The model under review builds one solid part; all positions refer to its coordinate system, in mm. A direction names the side the tool comes from. Give positions to 0.01 mm unless a question says otherwise; leave off trailing zeros. Loops run counter-clockwise (first coordinate to the right, second up) from the corner with the lowest first, then second, coordinate; pieces in that order, holes last. Notation, with made-up numbers: M -23.5,-7 L 28.5,-7 A18 ccw 28.5,20 Z; hole C -7,11.25 d4. An arc over 180 degrees is marked long. Return JSON: item names as keys, results as strings. Group by question number.
```python
from build123d import *

# Parameters (mm, degrees)
SKETCH1_W           = 20
SKETCH1_H           = 18
BOSS_EXTRUDE1_DEPTH = 25
SKETCH2_R           = 4
CUT_EXTRUDE1_DEPTH  = 26
CHAMFER1_SIZE       = 2
BOSS_EXTRUDE2_DEPTH = 1.5
CUT_EXTRUDE2_DEPTH  = 0.5
BOSS_EXTRUDE3_DEPTH = 40
SKETCH6_W           = 1
SKETCH6_H           = 1
CUT_EXTRUDE3_DEPTH  = 8


with BuildPart() as part:
    # Sketch1 → Boss-Extrude1 (new body)
    with BuildSketch(Plane.XY):
        Rectangle(SKETCH1_W, SKETCH1_H)
    extrude(amount=BOSS_EXTRUDE1_DEPTH)

    # Sketch2 → Cut-Extrude1 (cut, through all)
    with BuildSketch(Plane.XY.offset(25)):
        Circle(SKETCH2_R)
    extrude(amount=-CUT_EXTRUDE1_DEPTH, mode=Mode.SUBTRACT)

    # Chamfer1
    chamfer1_edges = [part.edges().sort_by_distance(p)[0] for p in [
        (10, 9, 12.5),
        (10, -9, 12.5),
        (-10, -9, 12.5),
        (-10, 9, 12.5),
    ]]
    chamfer(chamfer1_edges, length=CHAMFER1_SIZE)

    # Sketch3 → Boss-Extrude2 (add)
    with BuildSketch(Plane(origin=(0, 9, 0), x_dir=(1, 0, 0), z_dir=(0, 1, 0))):
        with BuildLine():
            Line((-7.418918919, -22.013513514), (-1.418918919, -4.513513514))
            ThreePointArc((-1.418918919, -4.513513514), (0.486486486, -3.581081081), (1.418918919, -5.486486486))
            Line((1.418918919, -5.486486486), (-4.581081081, -22.986486486))
            ThreePointArc((-4.581081081, -22.986486486), (-6.486486486, -23.918918919), (-7.418918919, -22.013513514))
        make_face()
    extrude(amount=BOSS_EXTRUDE2_DEPTH)

    # Sketch4 → Cut-Extrude2 (cut)
    with BuildSketch(Plane(origin=(0, 10.5, 0), x_dir=(1, 0, 0), z_dir=(0, 1, 0))):
        with BuildLine():
            Line((-6.945945946, -22.175675676), (-0.945945946, -4.675675676))
            ThreePointArc((-0.945945946, -4.675675676), (0.324324324, -4.054054054), (0.945945946, -5.324324324))
            Line((0.945945946, -5.324324324), (-5.054054054, -22.824324324))
            ThreePointArc((-5.054054054, -22.824324324), (-6.324324324, -23.445945946), (-6.945945946, -22.175675676))
        make_face()
    extrude(amount=-CUT_EXTRUDE2_DEPTH, mode=Mode.SUBTRACT)

    # Sketch5 → Boss-Extrude3 (add)
    with BuildSketch(Plane(origin=(0, 0, 0), x_dir=(-1, 0, 0), z_dir=(0, 0, -1))):
        Polygon((-10, 4), (-16, 4), (-17, 3), (-17, -3), (-16, -4), (-10, -4), align=None)
    extrude(amount=-BOSS_EXTRUDE3_DEPTH)

    # Sketch6 → Cut-Extrude3 (cut, through all)
    with BuildSketch(Plane.ZY.offset(-10)):
        with Locations((25.5, 3.5)):
            Rectangle(SKETCH6_W, SKETCH6_H)
        with Locations((27.25, 3.5)):
            Rectangle(SKETCH6_W, SKETCH6_H)
        with Locations((29, 3.5)):
            Rectangle(SKETCH6_W, SKETCH6_H)
        with Locations((30.75, 3.5)):
            Rectangle(SKETCH6_W, SKETCH6_H)
    extrude(amount=-CUT_EXTRUDE3_DEPTH, mode=Mode.SUBTRACT)


solid = part.part
```
(1) Add section B-B (z = 2.5). Write out the cut boundary in (x, y), and give its area (3 significant figures).
(2) Add section C-C (x = 15). Write out the cut boundary in (y, z), and give its area (3 significant figures).
(3) Add section A-A (y = 0). Write out the cut boundary in (x, z).
(4) Add section D-D (z = 37.5). Write out the cut boundary in (x, y).
(5) For pin 1 (0.8 mm diameter, centred on x = 15, z = 27, fed in from +Y); pin 2 (0.8 mm diameter, centred on x = 13.5, z = 29, fed in from +Y); pin 3 (6 mm diameter, centred on y = 8, z = 18.5, fed in from +X), all flat-tipped, find the tip position at first contact; note any pin that passes through.
(6) For faces 4 (the flat face through (13.5, 3.5, 26.75)), 5 (the flat face through (10, -6, 12)), 6 (the flat face through (0, 9, 12)), list the 3-axis set-ups (+Z, -Z, +X, -X, +Y, -Y) from which the entire face can be reached by the end or side of a thin tool; tool diameter is ignored.
(7) Mouldability with a two-part tool opening along Z and no side actions: class faces 1 (the flat face through (13.5, 3.5, 31.25)), 2 (the flat face through (13.5, 3.5, 30.25)), 3 (the flat face through (16.5, 3.5, 29.9)) as released by +Z, released by -Z, zero draft, split by the parting line, or undercut.
(8) For probe 1 along Y at (x, z) = (0, 7.5); probe 2 along Y at (x, z) = (0, 19.5); probe 3 along Y at (x, z) = (15.5, 15.5), list the stretches that pass through material, from the lowest coordinate up.
Verdict:
{
 "1": {"outline": "M -10,-7 L -8,-9 L 8,-9 L 10,-7 L 10,-4 L 16,-4 L 17,-3 L 17,3 L 16,4 L 10,4 L 10,7 L 8,9 L -8,9 L -10,7 Z; hole C 0,0 d8", "area": "357 mm²"},
 "2": {"outline": "M -4,0 L 4,0 L 4,25 L 3,25 L 3,26 L 4,26 L 4,26.75 L 3,26.75 L 3,27.75 L 4,27.75 L 4,28.5 L 3,28.5 L 3,29.5 L 4,29.5 L 4,30.25 L 3,30.25 L 3,31.25 L 4,31.25 L 4,40 L -4,40 Z", "area": "316 mm²"},
 "3": {"outline": "M -10,0 L -4,0 L -4,25 L -10,25 Z; M 4,0 L 17,0 L 17,40 L 10,40 L 10,25 L 4,25 Z"},
 "4": {"outline": "M 10,-4 L 16,-4 L 17,-3 L 17,3 L 16,4 L 10,4 Z"},
 "5": {"pin 1": "stops at y = 4", "pin 2": "stops at y = 3", "pin 3": "stops at x = 10"},
 "6": {"face 4": "+X, -X, +Y", "face 5": "+Z, -Z, +X, -Y", "face 6": "+Y"},
 "7": {"face 1": "undercut", "face 2": "undercut", "face 3": "zero draft"},
 "8": {"probe 1": "y = -9 to -4, 4 to 10", "probe 2": "y = -9 to -4, 4 to 9", "probe 3": "y = -4 to 4"}
}
